Geometry check sheet. Reference: the model listing, model coordinates, mm. Face numbers are marked on the shaded views. A direction names the side the tool comes from. Round coordinates to 2 decimals unless told otherwise and drop trailing zeros. Loops run counter-clockwise (first coordinate to the right, second up) from the corner with the lowest first, then second, coordinate; pieces in that order, holes last. Notation, with made-up numbers: M -17,20.25 L 36,20.25 A24 cw 36,38.25 Z; hole C -36.75,-30 d8. An arc over 180 degrees is marked long. Answer in a Markdown table with one row per item. Add a question column.
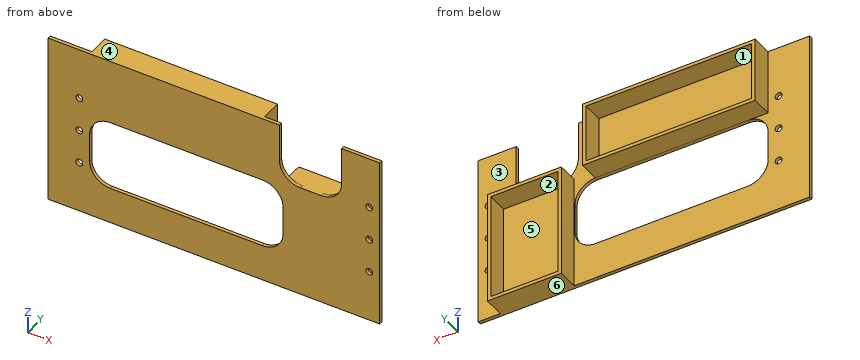
```python
from build123d import *

# Parameters (mm, degrees)
SKETCH1_W           = 450
SKETCH1_H           = 250
BOSS_EXTRUDE1_DEPTH = 5
CUT_EXTRUDE1_DEPTH  = 10
SKETCH3_W           = 250
SKETCH3_H           = 5
BOSS_EXTRUDE2_DEPTH = 30
SKETCH4_R           = 5
CUT_EXTRUDE2_DEPTH  = 30
SKETCH5_W           = 107
SKETCH5_H           = 165
SKETCH5_W_2         = 97
SKETCH5_H_2         = 155
SKETCH5_W_3         = 250
SKETCH5_H_3         = 95.00223246
SKETCH5_W_4         = 240
SKETCH5_H_4         = 85.00223246
BOSS_EXTRUDE3_DEPTH = 30


with BuildPart() as part:
    # Sketch1 → Boss-Extrude1 (new body)
    with BuildSketch(Plane(origin=(0, 0, 0), x_dir=(1, 0, 0), z_dir=(0, 1, 0))):
        Rectangle(SKETCH1_W, SKETCH1_H)
    extrude(amount=BOSS_EXTRUDE1_DEPTH)

    # Sketch2 → Cut-Extrude1 (cut)
    with BuildSketch(Plane(origin=(0, 5, 0), x_dir=(1, 0, 0), z_dir=(0, 1, 0))):
        with BuildLine():
            Line((-165, 72), (55, 72))
            ThreePointArc((55, 72), (76.213203436, 63.213203436), (85, 42))
            Line((85, 42), (85, 0))
            ThreePointArc((85, 0), (76.213203436, -21.213203436), (55, -30))
            Line((55, -30), (-165, -30))
            ThreePointArc((-165, -30), (-186.213203436, -21.213203436), (-195, 0))
            Line((-195, 0), (-195, 42))
            ThreePointArc((-195, 42), (-186.213203436, 63.213203436), (-165, 72))
        make_face()
        with BuildLine():
            Line((110, -40), (140, -40))
            ThreePointArc((140, -40), (161.213203436, -48.786796564), (170, -70))
            Line((170, -70), (170, -125))
            Line((170, -125), (80, -125))
            Line((80, -125), (80, -70))
            ThreePointArc((80, -70), (88.786796564, -48.786796564), (110, -40))
        make_face()
    extrude(amount=-CUT_EXTRUDE1_DEPTH, mode=Mode.SUBTRACT)

    # Sketch3 → Boss-Extrude2 (add)
    with BuildSketch(Plane.ZY.offset(225)):
        with Locations((0, 2.5)):
            Rectangle(SKETCH3_W, SKETCH3_H)
    extrude(amount=BOSS_EXTRUDE2_DEPTH)

    # Sketch4 → Cut-Extrude2 (cut)
    with BuildSketch(Plane(origin=(0, 5, 0), x_dir=(1, 0, 0), z_dir=(0, 1, 0))):
        with Locations((210, 0)):
            Circle(SKETCH4_R)
        with Locations((210, 50)):
            Circle(SKETCH4_R)
        with Locations((210, -50)):
            Circle(SKETCH4_R)
        with Locations((-210, -50)):
            Circle(SKETCH4_R)
        with Locations((-210, 0)):
            Circle(SKETCH4_R)
        with Locations((-210, 50)):
            Circle(SKETCH4_R)
    extrude(amount=-CUT_EXTRUDE2_DEPTH, mode=Mode.SUBTRACT)

    # Sketch5 → Boss-Extrude3 (add)
    with BuildSketch(Plane(origin=(0, 5, 0), x_dir=(1, 0, 0), z_dir=(0, 1, 0))):
        with Locations((139.576867422, 42.5)):
            Rectangle(SKETCH5_W, SKETCH5_H)
        with Locations((139.576867422, 42.5)):
            Rectangle(SKETCH5_W_2, SKETCH5_H_2, mode=Mode.SUBTRACT)
        with Locations((-69.634018269, -77.49888377)):
            Rectangle(SKETCH5_W_3, SKETCH5_H_3)
        with Locations((-69.634018269, -77.49888377)):
            Rectangle(SKETCH5_W_4, SKETCH5_H_4, mode=Mode.SUBTRACT)
    extrude(amount=BOSS_EXTRUDE3_DEPTH)


solid = part.part
```
1) Go/stop test with flat-tipped pins: pin 1 (2 mm diameter, centred on x = -37.5, y = 8, fed in from -Z); pin 2 (15 mm diameter, centred on y = 14.5, z = -21, fed in from -X); pin 3 (6 mm diameter, centred on y = 28.5, z = 84, fed in from +X). Record where each tip stops, or that it passes through.
2) Cross-section at D-D, the plane z = -99.5. Record the boundary of the cut face in (x, y).
3) Thickness scan on L1, parallel to Z at x = -210, y = 1.35; L2, parallel to Z at x = -130, y = 28; L3, parallel to X at y = 1.9, z = 50. Record the ranges inside material, lowest first. Write a range as [from, to].
4) Cross-section at A-A, the plane y = 20.5. Record the boundary of the cut face in (x, z), plus the area to 3 significant figures.
5) Cross-section at C-C, the plane z = 50. Record the boundary of the cut face in (x, y), plus the area to 3 significant figures.
6) Set-up check for the marked faces 5 and 6: record each of +Z, -Z, +X, -X, +Y, -Y from which the full face is reachable in a straight line by a thin tool's end or side.
7) Draft check along Z on the marked faces 1, 2, 3 and 4. Enter one of: +Z half, -Z half, draft (parallel to the pull), parting line (faces both ways), or undercut.
Worked answers:
| question | item | result |
|---|---|---|
| 1 | pin 1 | stops at z = 30 |
| 1 | pin 2 | stops at x = 86.08 |
| 1 | pin 3 | stops at x = 55.37 |
| 2 | outline | M -255,0 L 225,0 L 225,5 L 193.08,5 L 193.08,35 L 188.08,35 L 188.08,5 L 91.08,5 L 91.08,35 L 86.08,35 L 86.08,5 L -255,5 Z |
| 3 | L1 | z = [-125, -55], [-45, -5], [5, 45], [55, 125] |
| 3 | L2 | z = [30, 35], [120, 125] |
| 3 | L3 | x = [-255, -215], [-205, 87.64], [162.36, 205], [215, 225] |
| 4 | outline | M -194.63,30 L 55.37,30 L 55.37,125 L -194.63,125 Z; M 86.08,-125 L 193.08,-125 L 193.08,40 L 86.08,40 Z; hole M -189.63,35 L 50.37,35 L 50.37,120 L -189.63,120 Z; hole M 91.08,-120 L 188.08,-120 L 188.08,35 L 91.08,35 Z |
| 4 | area | 5,970 mm2 |
| 5 | outline | M -255,0 L -215,0 L -215,5 L -255,5 Z; M -205,0 L 87.64,0 L 87.64,5 L 55.37,5 L 55.37,35 L 50.37,35 L 50.37,5 L -189.63,5 L -189.63,35 L -194.63,35 L -194.63,5 L -205,5 Z; M 162.36,0 L 205,0 L 205,5 L 162.36,5 Z; M 215,0 L 225,0 L 225,5 L 215,5 Z |
| 5 | area | 2,230 mm2 |
| 6 | face 5 | +Y |
| 6 | face 6 | -Z, +X, -X, +Y, -Y |
| 7 | face 1 | undercut |
| 7 | face 2 | undercut |
| 7 | face 3 | draft |
| 7 | face 4 | +Z half |
